Autodesk Inventor part; units mm, degrees
ref_plane "YZ Plane" through (0, 0, 0) normal (1, 0, 0) x (0, 1, 0)
ref_plane "XZ Plane" through (0, 0, 0) normal (0, 1, 0) x (-1, 0, 0)
ref_plane "XY Plane" through (0, 0, 0) normal (0, 0, 1) x (1, 0, 0)
sketch "Sketch1" plane through (0, 0, 0) normal (0, 0, 1) x (1, 0, 0)
  line L0 (0, 0) -> (114.3, 0)
  line L1 (114.3, 0) -> (114.3, 228.6)
  line L2 (114.3, 228.6) -> (0, 228.6)
  line L3 (0, 228.6) -> (0, 0)
  dimension "d0" = 114.3
  dimension "d1" = 228.6
extrude "Extrusion1" add sketch "Sketch1" along normal blind 12.7
sketch "Sketch2" plane through (0, 0, 12.7) normal (0, 0, 1) x (1, 0, 0)
  point P0 (0, 0)
sketch "Sketch3" plane through (0, 0, 12.7) normal (0, 0, 1) x (1, 0, 0)
  line L0 (114.3, 0) -> (114.3, 228.6)
  line L1 (114.3, 228.6) -> (0, 354.1146)
  line L2 (0, 354.1146) -> (0, 228.6)
  line L3 (0, 228.6) -> (114.3, 228.6)
  point P0 (0, 0)
extrude "Extrusion2" add sketch "Sketch3" against normal blind 12.7
sketch "Sketch4" plane through (0, 0, 0) normal (0, 0, -1) x (-1, 0, 0)
  line L0 (0, 354.1146) -> (50.8, 354.1146)
  line L1 (50.8, 354.1146) -> (50.8, 176.3146)
  line L2 (50.8, 176.3146) -> (0, 176.3146)
  line L3 (0, 176.3146) -> (0, 354.1146)
  point P0 (0, 0)
  point P1 (0, 354.1146)
  dimension "d6" = 50.8
  dimension "d7" = 177.8
extrude "Extrusion3" add sketch "Sketch4" against normal blind 12.7
sketch "Sketch5" plane through (0, 0, 12.7) normal (0, 0, 1) x (1, 0, 0)
  line L0 (-50.8, 354.1146) -> (-50.8, 176.3146)
  line L1 (-50.8, 354.1146) -> (60.5424, 354.1146)
  line L2 (60.5424, 354.1146) -> (60.5424, 316.0146)
  line L3 (60.5424, 316.0146) -> (-50.8, 316.0146)
  line L4 (-50.8, 316.0146) -> (-50.8, 354.1146)
  point P0 (0, 0)
  dimension "d10" = 38.1
extrude "Extrusion4" cut sketch "Sketch5" against normal blind 25.4
properties part number "motor mount platform right side"
Check sheet for the modelled part. Datum: model origin and axes. Units: mm. A direction names the side the tool comes from. Coordinates: 2 decimals unless noted, no trailing zeros. Write each loop counter-clockwise with the first axis right and the second up, starting at its lowest first coordinate (ties: lowest second). Pieces come first, ordered by that corner, then holes. Notation, with made-up numbers: (6.25, 26) - (30.25, 26) arc R20 ccw to (30.25, 61) - close; hole circle Ø6 at (30, -40). An arc over 180 degrees is marked (long way). One line per question, with ' | ' between items.
Item 1: Access from +Z, -Z, +X, -X, +Y, -Y to the whole of each face (thin tool, end or side, straight path). Record for faces 1 (the face through (-50.8, 247, 6)), 2 (the face through (-26, 176.315, 6)).
Determined:
face 1: +Z, -Z, -X, +Y, -Y | face 2: +Z, -Z, -X, -Y
Item 2: Thickness scan on line 1 (X direction, y = 111.5, z = 12.25); line 2 (Y direction, x = -39.5, z = 10.75); line 3 (X direction, y = 287.5, z = 7). Record the ranges inside material, lowest first. Write a range as [from, to].
Determined:
line 1: x = [0, 114.3] | line 2: y = [176.31, 316.01] | line 3: x = [-50.8, 60.66]
Item 3: Sectioned sample at B-B on x = -11.5. Record the boundary of the cut face in (y, z).
Determined:
outline: (176.31, 0) - (316.01, 0) - (316.01, 12.7) - (176.31, 12.7) - close
Item 4: Sectioned sample at C-C on y = 20.5. Record the boundary of the cut face in (x, z), plus the area to 3 significant figures.
Determined:
outline: (0, 0) - (114.3, 0) - (114.3, 12.7) - (0, 12.7) - close | area: 1,450 mm2
Item 5: Gauge pin test, flat ends, axial feed: P1, Ø1.5, axis at y = 151, z = 2.5, coming from the -X side; P2, Ø3, axis at y = 240, z = 6.5, coming from the +X side; P3, Ø1.5, axis at x = 68, z = 4.5, coming from the +Y side. Record the tip position at first contact, or that the pin passes through.
Determined:
P1: stops at x = 0 | P2: stops at x = 105.28 | P3: stops at y = 280.27
Item 6: Sectioned sample at A-A on z = 4.75. Record the boundary of the cut face in (x, y), plus the area to 3 significant figures.
Determined:
outline: (-50.8, 176.31) - (0, 176.31) - (0, 0) - (114.3, 0) - (114.3, 228.6) - (34.7, 316.01) - (-50.8, 316.01) - close | area: 39,700 mm2
